```python
from build123d import *

# Parameters (mm, degrees)
BOSS_EXTRUDE1_DEPTH      = 5
BOSS_EXTRUDE1_DEPTH_BACK = 5
SKETCH1_R                = 10
SKETCH1_R_2              = 7.5


with BuildPart() as part:
    # Sketch1 → Boss-Extrude1 (new, two sides: drawn at the far end of the back side and taken through both)
    with BuildSketch(Plane.XY.offset(-BOSS_EXTRUDE1_DEPTH_BACK)):
        with BuildLine():
            Line((0.872093023, 14.974626999), (43.726744186, 12.478855832))
            ThreePointArc((43.726744186, 12.478855832), (55.5, 0), (43.726744186, -12.478855832))
            Line((43.726744186, -12.478855832), (0.872093023, -14.974626999))
            ThreePointArc((0.872093023, -14.974626999), (-15, 0), (0.872093023, 14.974626999))
        make_face()
        Circle(SKETCH1_R, mode=Mode.SUBTRACT)
        with Locations((43, 0)):
            Circle(SKETCH1_R_2, mode=Mode.SUBTRACT)
    extrude(amount=BOSS_EXTRUDE1_DEPTH + BOSS_EXTRUDE1_DEPTH_BACK)


solid = part.part
```
The listing builds one solid part. Answer for the finished solid, in the listing's coordinates (mm). Give positions to 0.01 mm unless a question says otherwise; leave off trailing zeros. Order: outer loops, then holes, each group sorted by start corner. A loop starts at its lowest first (then second) coordinate and runs counter-clockwise, first axis right, second up. Notation, with made-up numbers: (74, 23) -> (101, 23) arc R16 ccw to (101, 38) -> close; hole circle Ø5 at (-25, -14.75). An arc over 180 degrees is marked (long way). One line per item, written item: value.
1) Find the intervals of material crossed by line 1 (X direction, y = 5.5, z = 3); line 2 (X direction, y = 4.75, z = 2); line 3 (Y direction, x = 43, z = -2), in increasing order.
Reported:
line 1: x = -13.96 to -8.35, 8.35 to 37.9, 48.1 to 54.22
line 2: x = -14.23 to -8.8, 8.8 to 37.2, 48.8 to 54.56
line 3: y = -12.52 to -7.5, 7.5 to 12.52
2) Find section A-A, the plane x = 0. Determine the outline of the cut face in (y, z).
Reported:
outline: (-15, -5) -> (-10, -5) -> (-10, 5) -> (-15, 5) -> close; (10, -5) -> (15, -5) -> (15, 5) -> (10, 5) -> close
3) Find section D-D, the plane x = 43. Determine the outline of the cut face in (y, z).
Reported:
outline: (-12.52, -5) -> (-7.5, -5) -> (-7.5, 5) -> (-12.52, 5) -> close; (7.5, -5) -> (12.52, -5) -> (12.52, 5) -> (7.5, 5) -> close
4) Flat-ended cylindrical pins translate along their axes: P1, Ø5, axis at x = 23, z = -0.5, coming from the -Y side; P2, Ø6, axis at y = -4.5, z = -0.5, coming from the +X side; P3, Ø1, axis at y = 10, z = 3, coming from the +X side; P4, Ø9, axis at x = 43, y = 0, coming from the -Z side. Find the tip coordinate at first contact, or state that the pin passes through.
Reported:
P1: stops at y = -13.83
P2: stops at x = 55.41
P3: stops at x = 51.12
P4: passes through
5) Determine the mould class of faces 1 (the flat face through (21, 0, -5)), 2 (the flat face through (21.999, 13.744, -0.07)), 3 (the cylindrical face through (50.154, 2.253, -0.07)) for opening direction X: pulls with the +X half, pulls with the -X half, needs draft (parallel to the pull), parting line crosses it, or undercut.
Reported:
face 1: needs draft
face 2: pulls with the +X half
face 3: undercut
6) Find section C-C, the plane z = -3.5. Determine the outline of the cut face in (x, y).
Reported:
outline: (0.87, -14.97) -> (43.73, -12.48) arc R12.5 ccw to (43.73, 12.48) -> (0.87, 14.97) arc R15 ccw (long way) to start; hole circle Ø20 at (0, 0); hole circle Ø15 at (43, 0)
7) Find section B-B, the plane y = 0. Determine the outline of the cut face in (x, z), plus the area to 3 significant figures.
Reported:
outline: (-15, -5) -> (-10, -5) -> (-10, 5) -> (-15, 5) -> close; (10, -5) -> (35.5, -5) -> (35.5, 5) -> (10, 5) -> close; (50.5, -5) -> (55.5, -5) -> (55.5, 5) -> (50.5, 5) -> close
area: 355 mm^2
